Autodesk Inventor part; units mm, degrees
ref_plane "Start plane" through (0, 0, 0) normal (0, 0, 1) x (1, 0, 0)
ref_plane "End plane" through (0, 0, 800.1) normal (0, 0, 1) x (1, 0, 0)
ref_plane "Work Plane4" through (0, 53.34, 800.1) normal (0, -1, 0) x (1, 0, 0)
ref_plane "Start plane" through (0, 0, 0) normal (0, 0, 1) x (1, 0, 0)
ref_plane "End plane" through (0, 0, 800.1) normal (0, 0, 1) x (1, 0, 0)
sketch "Sketch" plane through (0, 0, 0) normal (0, 0, 1) x (1, 0, 0)
  circle A0 centre (0, 0) radius 13.3223
  circle A1 centre (0, 0) radius 16.7005
  dimension "d0" = 33.401
  dimension "d1" = 3.3782
extrude "Body" add sketch "Sketch" along normal up to surface (800.1 mm away) from surface at 0
sketch "Sketch3" plane through (0, 0, 0) normal (0, 0, 1) x (1, 0, 0)
  line L0 (0, 0) -> (10, 0)
ref_plane "Work Plane3" through (0, 0, 0) normal (0, -1, 0) x (1, 0, 0)
sketch "Sketch4" plane through (0, 0, 0) normal (0, -1, 0) x (1, 0, 0)
  line L0 (-2, 0) -> (12, 0)
  line L1 (-2, 800.1) -> (12, 800.1)
  dimension "d7" = 800.1
ref_plane "Work Plane4" through (0, 53.34, 800.1) normal (0, -1, 0) x (1, 0, 0)
ref_plane "Work Plane5" through (0, -22.86, 800.1) normal (0, -1, 0) x (1, 0, 0)
ref_plane "Work Plane6" through (0, 15.24, 800.1) normal (0, -1, 0) x (1, 0, 0)
sketch "Sketch5" plane through (0, 15.24, 800.1) normal (0, -1, 0) x (1, 0, 0)
  circle A0 centre (0, 0) radius 21.082
  circle A1 centre (0, 0) radius 17.526
extrude "Extrusion2" cut sketch "Sketch5" along normal up to surface (76.2 mm away) from surface at -38.1 contours A0 | A1
ref_plane "Work Plane7" through (16.7005, 0, 0) normal (1, 0, 0) x (0, 1, 0)
sketch "Sketch6" plane through (16.7005, 0, 0) normal (1, 0, 0) x (0, 1, 0)
  arc A0 (15.4462, 6.35) -> (-15.4462, 6.35) centre (0, 0) ccw
  line L0 (-16.7005, 0) -> (16.7005, 0)
  arc A1 (16.7005, 0) -> (-16.7005, 0) centre (0, 0) ccw
  point P0 (0, 0)
extrude "Extrusion3" cut sketch "Sketch6" against normal through all
ref_plane "Work Plane8" through (0, 16.7005, 0) normal (0, 1, 0) x (-1, 0, 0)
sketch "Sketch7" plane through (0, 16.7005, 0) normal (0, 1, 0) x (-1, 0, 0)
  line L0 (0, 0) -> (-16.7005, 16.7005)
  line L1 (16.7005, 16.7005) -> (0, 0)
  line L2 (-6.35, 6.35) -> (6.35, 6.35)
  dimension "d12" = 6.35
extrude "Extrusion4" cut sketch "Sketch7" against normal through all
equation "\"d0\" = G_H"
equation "\"d1\" = G_T"
equation "\"d2\" = G_L"
equation "\"G_H\" = 33.401"
equation "\"G_T\" = 3.3782"
equation "\"G_L\" = d7"
equation "\"G_OFFSET_START\" = 0"
equation "\"G_OFFSET_END\" = 0"
equation "\"d5\" = G_OFFSET_END + B_L"
equation "\"B_L\" = 800.1"
properties part number "ANSI - 1 x 0.133 - 31.5" material "Aluminum 6061"
Part model, mm, in its own coordinate system. Give positions to 0.01 mm unless a question says otherwise; leave off trailing zeros. Order: outer loops, then holes, each group sorted by start corner. A loop starts at its lowest first (then second) coordinate and runs counter-clockwise, first axis right, second up. Notation, with made-up numbers: (-13, 61) - (24, 61) arc R33 ccw to (24, 98) - close; hole circle Ø3 at (-31, 28.25). An arc over 180 degrees is marked (long way). Use one line per item in the form item = value.
Item 1: Slice it at C-C on z = 582.5. Give the cut face in (x, y), and give its area (3 significant figures).
Solution:
outline = circle Ø33.4 at (0, 0); hole circle Ø26.64 at (0, 0)
area = 319 mm2
Item 2: Pin check, flat tips, straight feed: pin 1 Ø8 at (x, z) = (10.5, 266.5) entering from -Y; pin 2 Ø3 at (x, z) = (-12, 684.5) entering from +Y; pin 3 Ø2 at (y, z) = (11.5, 443.5) entering from +X. Stop position of each tip, or through.
Solution:
pin_1 = -15.38
pin_2 = 12.99
pin_3 = 12.99
Item 3: Probe probe 1 along X at (y, z) = (0, 239); probe 2 along X at (y, z) = (10.5, 554.5). List the from-to ranges inside material, lowest first. Write a range as from..to.
Solution:
probe_1 = -16.7..-13.32, 13.32..16.7
probe_2 = -12.99..-8.2, 8.2..12.99
Item 4: Two-plate mould, pull along X, no slides. Class faces 1 (the face through (-11.998, -6.109, 782.765)), 2 (the face through (-3.62, 16.303, 391.327)): released by +X, released by -X, zero draft, split by the parting line, or undercut.
Solution:
face_1 = undercut
face_2 = split by the parting line
Item 5: Slice it at A-A on y = 0. Give the cut face in (x, z).
Solution:
outline = (-16.7, 16.7) - (-13.32, 16.7) - (-13.32, 783.76) arc R21.08 cw to (-16.7, 787.23) - close; (13.32, 16.7) - (16.7, 16.7) - (16.7, 787.23) arc R21.08 cw to (13.32, 783.76) - close
Item 6: Slice it at B-B on x = 0. Give the cut face in (y, z).
Solution:
outline = (-16.7, 6.35) - (-15.45, 6.35) arc R16.7 cw to (-13.32, 10.07) - (-13.32, 779.02) - (-16.7, 779.02) - close; (13.32, 10.07) arc R16.7 cw to (15.45, 6.35) - (16.7, 6.35) - (16.7, 779.02) - (13.32, 779.02) - close
